Here's the drawing with two shaded views (mm, measured from the low corner). I have some questions. Give positions to 0.01 mm unless a question says otherwise; leave off trailing zeros. Loops run counter-clockwise (first coordinate to the right, second up) from the corner with the lowest first, then second, coordinate; pieces in that order, holes last. Notation, with made-up numbers: (17, 20.5) - (44, 20.5) arc R32 ccw to (44, 57.5) - close; hole circle Ø1 at (86.5, 83.25). An arc over 180 degrees is marked (long way). Answer as a JSON object with one key per item and string values. Group by question number.
Item 1: Please list where these lines run through material, in increasing order: L1, parallel to Y at x = 38.1, z = 1.45; L2, parallel to X at y = 12.5, z = 1.3; L3, parallel to Y at x = 12, z = 1.75.
Item 2: Suppose I cut it at D-D on y = 62.5. Write out the boundary of the cut face in (x, z) (1 decimal).
Item 3: Suppose I cut it at A-A on y = 38.1. Write out the boundary of the cut face in (x, z) (1 decimal).
Item 4: Suppose I cut it at C-C on x = 14.5. Write out the boundary of the cut face in (y, z) (1 decimal).
Item 5: Suppose I cut it at B-B on x = 38.1. Write out the boundary of the cut face in (y, z) (1 decimal).
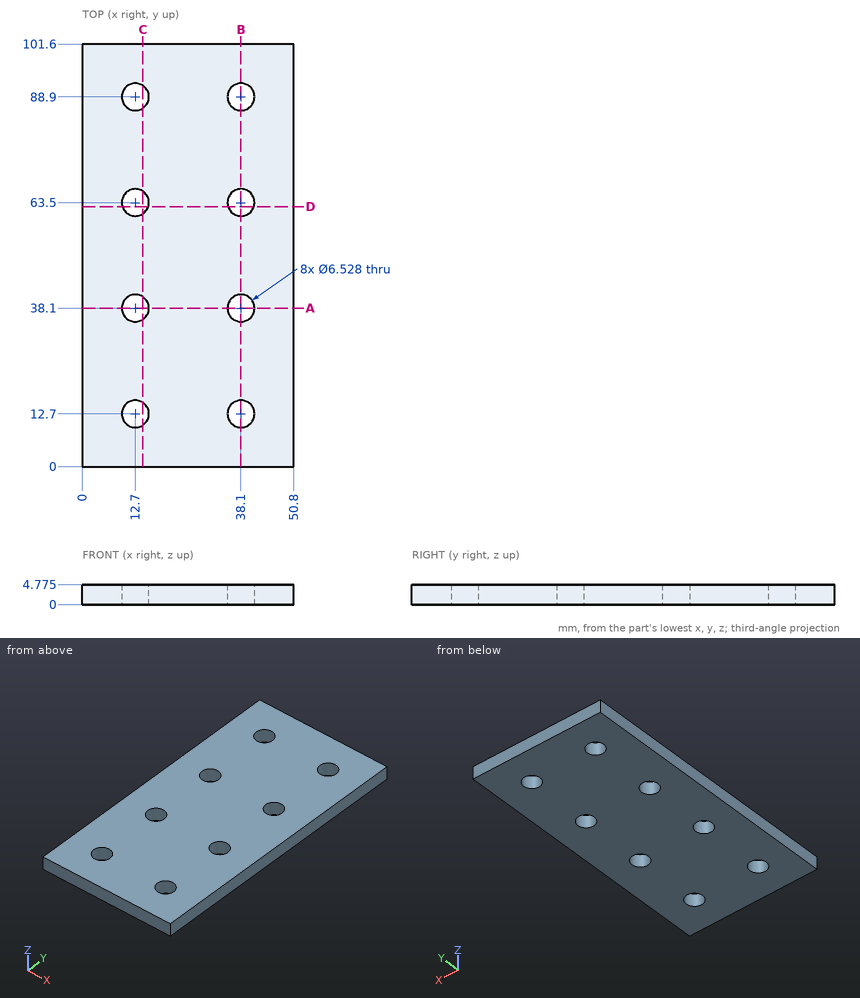
Worked out:
{
 "1": {"L1": "y = 0 to 9.44, 15.96 to 34.84, 41.36 to 60.24, 66.76 to 85.64, 92.16 to 101.6", "L2": "x = 0 to 9.44, 15.96 to 34.84, 41.36 to 50.8", "L3": "y = 0 to 9.51, 15.89 to 34.91, 41.29 to 60.31, 66.69 to 85.71, 92.09 to 101.6"},
 "2": {"outline": "(0, 0) - (9.6, 0) - (9.6, 4.8) - (0, 4.8) - close; (15.8, 0) - (35, 0) - (35, 4.8) - (15.8, 4.8) - close; (41.2, 0) - (50.8, 0) - (50.8, 4.8) - (41.2, 4.8) - close"},
 "3": {"outline": "(0, 0) - (9.4, 0) - (9.4, 4.8) - (0, 4.8) - close; (16, 0) - (34.8, 0) - (34.8, 4.8) - (16, 4.8) - close; (41.4, 0) - (50.8, 0) - (50.8, 4.8) - (41.4, 4.8) - close"},
 "4": {"outline": "(0, 0) - (10, 0) - (10, 4.8) - (0, 4.8) - close; (15.4, 0) - (35.4, 0) - (35.4, 4.8) - (15.4, 4.8) - close; (40.8, 0) - (60.8, 0) - (60.8, 4.8) - (40.8, 4.8) - close; (66.2, 0) - (86.2, 0) - (86.2, 4.8) - (66.2, 4.8) - close; (91.6, 0) - (101.6, 0) - (101.6, 4.8) - (91.6, 4.8) - close"},
 "5": {"outline": "(0, 0) - (9.4, 0) - (9.4, 4.8) - (0, 4.8) - close; (16, 0) - (34.8, 0) - (34.8, 4.8) - (16, 4.8) - close; (41.4, 0) - (60.2, 0) - (60.2, 4.8) - (41.4, 4.8) - close; (66.8, 0) - (85.6, 0) - (85.6, 4.8) - (66.8, 4.8) - close; (92.2, 0) - (101.6, 0) - (101.6, 4.8) - (92.2, 4.8) - close"}
}
